Source: three-view drawing plus pictorial views. Frame: mm from the lowest corner of the part. Give positions to 0.01 mm unless a question says otherwise; leave off trailing zeros. Loops run counter-clockwise (first coordinate to the right, second up) from the corner with the lowest first, then second, coordinate; pieces in that order, holes last. Notation, with made-up numbers: M 16,15.5 L 57,15.5 A20 ccw 57,20.5 Z; hole C 12.25,82 d3. An arc over 180 degrees is marked long. Write item = value, one per line.
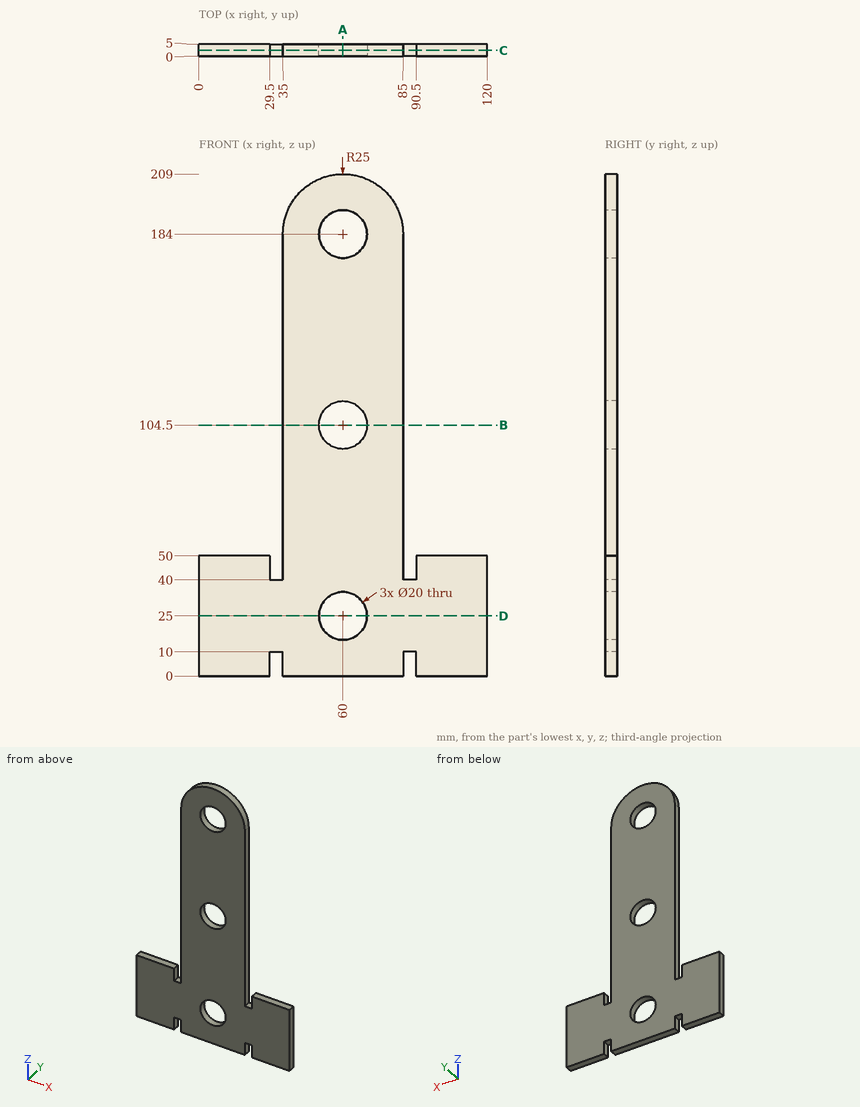
1. Cut plane D-D, the plane z = 25. Return the cut outline in (x, y).
Derived:
outline = M 0,0 L 50,0 L 50,5 L 0,5 Z; M 70,0 L 120,0 L 120,5 L 70,5 Z
2. Material intervals for probe 1 along Z at (x, y) = (60, 1.8); probe 2 along Z at (x, y) = (53, 0.95); probe 3 along X at (y, z) = (3.95, 25), sorted ascending. Write a range as from..to.
Derived:
probe_1 = 0..15, 35..94.5, 114.5..174, 194..209
probe_2 = 0..17.86, 32.14..97.36, 111.64..176.86, 191.14..208
probe_3 = 0..50, 70..120
3. Cut plane C-C, the plane y = 2.35. Return the cut outline in (x, z).
Derived:
outline = M 0,0 L 29.5,0 L 29.5,10 L 35,10 L 35,0 L 85,0 L 85,10 L 90.5,10 L 90.5,0 L 120,0 L 120,50 L 90.5,50 L 90.5,40 L 85,40 L 85,184 A25 ccw 35,184 L 35,40 L 29.5,40 L 29.5,50 L 0,50 Z; hole C 60,25 d20; hole C 60,104.5 d20; hole C 60,184 d20
4. Cut plane B-B, the plane z = 104.5. Return the cut outline in (x, y).
Derived:
outline = M 35,0 L 50,0 L 50,5 L 35,5 Z; M 70,0 L 85,0 L 85,5 L 70,5 Z
5. First-contact query: pin 1 Ø3 at (y, z) = (4, 109) entering from +X; pin 2 Ø1.5 at (x, y) = (86.5, 1.5) entering from +Z; pin 3 Ø1.5 at (x, y) = (87, 2) entering from -Z; pin 4 Ø16 at (x, z) = (60, 104.5) entering from +Y. Flat tips, straight axial feed; report the tip coordinate or a pass-through.
Derived:
pin_1 = 85
pin_2 = 40
pin_3 = 10
pin_4 = through
6. Cut plane A-A, the plane x = 60. Return the cut outline in (y, z).
Derived:
outline = M 0,0 L 5,0 L 5,15 L 0,15 Z; M 0,35 L 5,35 L 5,94.5 L 0,94.5 Z; M 0,114.5 L 5,114.5 L 5,174 L 0,174 Z; M 0,194 L 5,194 L 5,209 L 0,209 Z
